Autodesk Inventor part; units mm, degrees
ref_plane "YZ Plane" through (0, 0, 0) normal (1, 0, 0) x (0, 1, 0)
ref_plane "XZ Plane" through (0, 0, 0) normal (0, 1, 0) x (-1, 0, 0)
ref_plane "XY Plane" through (0, 0, 0) normal (0, 0, 1) x (1, 0, 0)
sketch "Sketch1" plane through (0, 0, 0) normal (0, 1, 0) x (-1, 0, 0)
  line L0 (0, 121.25) -> (0, 121.25)
  line L1 (32, 89.25) -> (32, -89.25)
  line L2 (0, -121.25) -> (0, -121.25)
  line L3 (-32, -89.25) -> (-32, 89.25)
  line L4 (32, 0) -> (-32, 0) construction
  arc A0 (32, 89.25) -> (0, 121.25) centre (0, 89.25) ccw
  arc A1 (0, 121.25) -> (-32, 89.25) centre (0, 89.25) ccw
  arc A2 (0, -121.25) -> (32, -89.25) centre (0, -89.25) ccw
  arc A3 (-32, -89.25) -> (0, -121.25) centre (0, -89.25) ccw
  arc A4 (0, -136.25) -> (47, -89.25) centre (0, -89.25) ccw
  line L5 (47, -89.25) -> (47, 89.25)
  arc A5 (47, 89.25) -> (-34.4238, 121.25) centre (0, 89.25) ccw
  arc A6 (-34.4238, 121.25) -> (-47, 89.25) centre (0, 89.25) ccw
  line L6 (-47, 89.25) -> (-47, -89.25)
  arc A7 (-47, -89.25) -> (0, -136.25) centre (0, -89.25) ccw
  arc A8 (0, 129.25) -> (-40, 89.25) centre (0, 89.25) ccw construction
  line L7 (-40, 89.25) -> (-40, -89.25) construction
  arc A9 (-40, -89.25) -> (24, -121.25) centre (0, -89.25) ccw construction
  arc A10 (24, -121.25) -> (40, -89.25) centre (0, -89.25) ccw construction
  line L8 (40, -89.25) -> (40, 89.25) construction
  arc A11 (40, 89.25) -> (0, 129.25) centre (0, 89.25) ccw construction
  circle A12 centre (0, -129.25) radius 2.05
  circle A13 centre (0, 129.25) radius 2.05
  circle A14 centre (-39.9488, 91.2737) radius 2.05
  circle A15 centre (39.9488, 91.2737) radius 2.05
  circle A16 centre (-40, 30.42) radius 2.05
  circle A17 centre (40, 30.42) radius 2.05
  circle A18 centre (0, -129.25) radius 2.05
  circle A19 centre (-39.9488, -91.2737) radius 2.05
  circle A20 centre (39.9488, -91.2737) radius 2.05
  circle A21 centre (-40, -30.42) radius 2.05
  circle A22 centre (40, -30.42) radius 2.05
  circle A23 centre (0, 121.25) radius 5
  circle A24 centre (0, -121.25) radius 5
  point P0 (0, 0)
  point P1 (32, -121.25)
  point P2 (32, 121.25)
  point P3 (-32, -121.25)
  point P4 (0, 0)
  point P5 (-40, 0)
  point P6 (40, 0)
  point P7 (4.9847, -120.8594)
  point P8 (-4.9847, -120.8594)
  point P9 (0, -121.25)
  point P10 (-4.9847, 120.8594)
  point P11 (4.9847, 120.8594)
  point P12 (0, 121.25)
  dimension "d0" = 242.5
  dimension "d1" = 64
  dimension "d2" = 32
  dimension "d3" = 32
  dimension "d4" = 15
  dimension "d5" = 8
  dimension "d6" = 4.1
  dimension "d7" = 4.1
  dimension "d10" = 87.1
  dimension "d14" = 87.1
  dimension "d16" = 4.1
  dimension "d17" = 30.42
  dimension "d18" = 4.1
  dimension "d19" = 30.42
  dimension "d20" = 10
  dimension "d21" = 10
extrude "Extrusion1" add sketch "Sketch1" against normal blind 3 contours L1 A2 A24 A3 L3 A1 A23 A0 | A23 A1 A0 | A0 A1 A23 | A24 A3 A2 | A2 A3 A24 | A7 L6 A6 A5 L5 A4
extrude "Extrusion2" add sketch "Sketch1" along normal blind 3 contours A23 A1 A0 | A2 A3 A24 picked at (0.9662, 119.6201) picked at (0.9662, -119.6201)
properties part number "top_housing_base-plate"
Read the model definition and answer for the solid it produces. Units are mm, in the model's axes. Round coordinates to 2 decimals unless told otherwise and drop trailing zeros. Order: outer loops, then holes, each group sorted by start corner. A loop starts at its lowest first (then second) coordinate and runs counter-clockwise, first axis right, second up.
1) The part is cut by section A-A on z = -7.5. Write down the section's boundary in (x, y), plus the area to 3 significant figures.
2) Flat-ended cylindrical pins translate along their axes: pin 1 (10 mm diameter, centred on x = 19, z = -21.5, fed in from +Y); pin 2 (2.5 mm diameter, centred on x = -40, z = -30.42, fed in from +Y); pin 3 (1 mm diameter, centred on x = 15, y = -2.5, fed in from +Z). Find the tip coordinate at first contact, or state that the pin passes through.
3) The mould has two halves that part along Z. Classify faces 1 (the face through (0.1, 1.48, -116.25)), 2 (the face through (1.03, -1.48, -136.24)), 3 (the face through (-0.1, 1.48, 116.25)), 4 (the face through (43.652, -1.479, 106.67)): released by +Z, released by -Z, zero draft, split by the parting line, or undercut.
4) Straight lines are drawn through the part: L1, parallel to Z at x = 40, y = -1; L2, parallel to Z at x = -38.5, y = -0.1; L3, parallel to Y at x = 11, z = 94.5. For each, find the intervals that lie inside material, in ascending order.
5) The part is cut by section B-B on x = -24.5. Write down the section's boundary in (y, z), plus the area to 3 significant figures.
Resolved:
1. outline: (-47, -3) - (47, -3) - (47, 0) - (-47, 0) - close
1. area: 282 mm2
2. pin 1: stops at y = 0
2. pin 2: passes through
2. pin 3: stops at z = 133.96
3. face 1: undercut
3. face 2: released by -Z
3. face 3: undercut
3. face 4: released by +Z
4. L1: z = -113.93 to -93.32, -89.22 to -32.47, -28.37 to 28.37, 32.47 to 89.22, 93.32 to 113.93
4. L2: z = -116.21 to -92.72, -89.82 to -31.82, -29.02 to 29.02, 31.82 to 89.82, 92.72 to 116.21
4. L3: y = -3 to 0
5. outline: (-3, -129.36) - (0, -129.36) - (0, 129.36) - (-3, 129.36) - close
5. area: 776 mm2
